Design review of the part built by this model. Coordinates are the model's own, in mm. A direction names the side the tool comes from. Round coordinates to 2 decimals unless told otherwise and drop trailing zeros. Order: outer loops, then holes, each group sorted by start corner. A loop starts at its lowest first (then second) coordinate and runs counter-clockwise, first axis right, second up. Notation, with made-up numbers: (43.25, 85) - (76.25, 85) arc R20 cw to (76.25, 112) - close; hole circle Ø9 at (89, 66). An arc over 180 degrees is marked (long way). Write item = value, one per line.
Autodesk Fusion 360 part; units mm, degrees
sketch "Sketch4" plane through (0, 0, 0) normal (0, 0, 1) x (1, 0, 0)
  line L0 (-17.0224, 4.5069) -> (-7.2135, 4.5755)
  line L1 (-6.882, 4.6055) -> (-0.9889, 5.6389)
  line L2 (-18, 0) -> (-17.9997, 1.25) construction
  line L3 (-17.9997, 1.25) -> (-18.0154, 3.5)
  line L4 (-18, 0) -> (-18, -0.25) construction
  line L5 (-18, -0.25) -> (-3.9671, -0.25)
  line L6 (-17.9997, 1.25) -> (-3.7746, 1.2463)
  arc A0 (2.7555, 5.0182) -> (-0.9889, 5.6389) centre (0, 0) ccw
  arc A1 (-3.9671, -0.25) -> (-3.7746, 1.2463) centre (0, 0) ccw
  line L7 (-18, -0.25) -> (-18, -10)
  line L8 (-15, -13) -> (9, -13)
  line L9 (12, -10) -> (12, -1.8332)
  line L10 (10.444, 0.7965) -> (2.7555, 5.0182)
  arc A2 (-7.2135, 4.5755) -> (-6.882, 4.6055) centre (-7.2274, 6.5754) ccw
  arc A3 (-7.2135, 4.5755) -> (-6.882, 4.6055) centre (-7.2274, 6.5754) ccw
  arc A4 (12, -1.8332) -> (10.444, 0.7965) centre (9, -1.8332) ccw
  arc A5 (9, -13) -> (12, -10) centre (9, -10) ccw
  arc A6 (-18, -10) -> (-15, -13) centre (-15, -10) ccw
  arc A7 (-17.0224, 4.5069) -> (-18.0154, 3.5) centre (-17.0154, 3.507) ccw
  point P0 (-18.0224, 4.4999)
  dimension "d18" = 7.95
  dimension "d22" = 18
  dimension "d24" = 4.5
  dimension "d26" = 1.25
  dimension "d27" = 0.25
  dimension "d28" = 2
  dimension "d29" = 3
  dimension "d30" = 3
  dimension "d31" = 1
  dimension "d56" = 1.75
extrude "Extrude2" add sketch "Sketch4" along normal blind 10 makes body 1
sketch "Sketch5" plane through (-0.0323, 4.6256, 0) normal (-0.007, 1, 0) x (-1, -0.007, 0)
  line L0 (7.1813, 0) -> (16.9905, 0)
  line L1 (16.9905, 0) -> (16.9905, 10)
  line L2 (16.9905, 10) -> (7.1813, 10)
  line L3 (7.1813, 10) -> (7.1813, 0)
  line L4 (12.0859, 10) -> (12.0859, 0) construction
  line L5 (16.9905, 5) -> (7.1813, 5) construction
hole "Hole2" at (-12.1179, 4.5412, 5) direction (0.007, -1, 0) diameter 3 end through all counterbore diameter 6 counterbore depth 2 bodies 1 1
sketch "Sketch6" plane through (0, 0, 10) normal (0, 0, 1) x (-1, 0, 0)
  line L0 (7.2135, -4.5755) -> (17.0224, -4.5069)
  arc A0 (17.0224, -4.5069) -> (18.0154, -3.5) centre (17.0154, -3.507) ccw
  line L1 (18.0154, -3.5) -> (17.9997, -1.25)
  line L2 (17.9997, -1.25) -> (3.7746, -1.2463)
  arc A1 (3.9671, 0.25) -> (3.7746, -1.2463) centre (0, 0) ccw
  line L3 (3.9671, 0.25) -> (18, 0.25)
  line L4 (18, 0.25) -> (18, 10)
  arc A2 (18, 10) -> (15, 13) centre (15, 10) ccw
  line L5 (15, 13) -> (-9, 13)
  arc A3 (-9, 13) -> (-12, 10) centre (-9, 10) ccw
  line L6 (-12, 10) -> (-12, 1.8332)
  arc A4 (-12, 1.8332) -> (-10.444, -0.7965) centre (-9, 1.8332) ccw
  line L7 (-10.444, -0.7965) -> (-2.7555, -5.0182)
  arc A5 (-2.7555, -5.0182) -> (0.9889, -5.6389) centre (0, 0) ccw
  line L8 (0.9889, -5.6389) -> (6.882, -4.6055)
  arc A6 (7.2135, -4.5755) -> (6.882, -4.6055) centre (7.2274, -6.5754) ccw
  line L9 (0, 0) -> (0, 3.975) construction
  line L10 (0, 3.975) -> (-12, 3.975) construction
  line L11 (-12, 3.975) -> (-12, 12.975) construction
  line L12 (-12, 8.475) -> (18, 8.475) construction
  line L13 (0, 3.975) -> (0, 13) construction
  line L14 (7, 8.475) -> (7, 6.4233) construction
  point P0 (-7, 8.475)
  point P1 (7, 8.475)
  dimension "d39" = 9
  dimension "d54" = 14
  dimension "d55" = 7
hole "Hole3" at (7, -8.475, 10) direction (0, 0, -1) diameter 3 end through all counterbore diameter 6 counterbore depth 3 bodies 1 1
hole "Hole4" at (-7, -8.475, 10) direction (0, 0, -1) diameter 3 end through all counterbore diameter 6 counterbore depth 3 bodies 1 1
sketch "Sketch7" plane through (-18, 0, 0) normal (-1, 0, 0) x (0, -1, 0)
  line L0 (0.25, 0) -> (10, 0)
  line L1 (10, 0) -> (10, 10)
  line L2 (10, 10) -> (0.25, 10)
  line L3 (0.25, 10) -> (0.25, 0)
  line L4 (5.125, 10) -> (5.125, 0) construction
  line L5 (10, 5) -> (0.25, 5) construction
  line L6 (6, 7.875) -> (4.25, 7.875)
  line L7 (4.25, 7.875) -> (4.25, 2.125)
  line L8 (4.25, 2.125) -> (6, 2.125)
  line L9 (6, 2.125) -> (6, 7.875)
  line L10 (6, 7.875) -> (4.25, 2.125) construction
  line L11 (4.25, 7.875) -> (6, 2.125) construction
  point P0 (5.125, 5)
  dimension "d50" = 1.75
  dimension "d51" = 5.75
extrude "Extrude3" cut sketch "Sketch7" against normal blind 8.81 contours L6 L7 L8 L9 bodies 1
copy_body "Body->Comp1" bodies 1 removing the originals makes body 2 in component "Guide Rail Clamp 1st Direction"
component "Guide Rail Clamp 1st Direction" placed x (1, 0, 0) y (0, 1, 0) z (0, 0, 1) at (0, 0, 0)
Item 1: The part is to be moulded in two halves that separate along Y. For faces 1 (the face through (8.33, -9.17, 3.45)), 2 (the face through (12, -6, 5)), 3 (the face through (11.14, -12.1, 4.93)), say which applies: +Y half, -Y half, draft (parallel to the pull), parting line (faces both ways), or undercut.
Data:
face_1 = undercut
face_2 = draft
face_3 = -Y half
Item 2: For faces 4 (the face through (-11.445, -9.545, 6.386)), 5 (the face through (-10, -0.25, 5)), 6 (the face through (-7.132, -5.478, 8.479)), list the 3-axis set-ups (+Z, -Z, +X, -X, +Y, -Y) from which the entire face can be reached by the end or side of a thin tool; tool diameter is ignored.
Data:
face_4 = none
face_5 = +Z, -Z, -X
face_6 = +Z
Item 3: Take a section at A-A, the plane x = 7. State the section outline as (y, z) points (3 decimals).
Data:
outline = (-13, 0) - (-9.975, 0) - (-9.975, 7) - (-11.475, 7) - (-11.475, 10) - (-13, 10) - close; (-6.975, 0) - (2.688, 0) - (2.688, 10) - (-5.475, 10) - (-5.475, 7) - (-6.975, 7) - close
Item 4: Take a section at D-D, the plane x = 2. State the section outline as (y, z) points.
Data:
outline = (-13, 0) - (-3.44, 0) - (-3.44, 10) - (-13, 10) - close; (3.44, 0) - (5.36, 0) - (5.36, 10) - (3.44, 10) - close
Item 5: Insertion check: P1, Ø0.5, axis at x = -12, y = -5.5, coming from the -Z side; P2, Ø1.4, axis at y = -5.5, z = 6, coming from the -X side; P3, Ø3.5, axis at x = 7, y = -8.475, coming from the +Z side; P4, Ø3, axis at x = -14.5, z = 3.5, coming from the +Y side. Each pin has a flat end and moves straight along its axis. Give the tip position at first contact, or say it passes through.
Data:
P1 = 0
P2 = -18
P3 = 7
P4 = 4.53
Item 6: For line 1 along Y through (x, z) = (-14.5, 6); line 2 along Y through (x, z) = (-4.5, 1.5); line 3 along X through (y, z) = (-3.5, 4), list the stretches that pass through material, from the lowest coordinate up. Write a range as [from, to].
Data:
line_1 = [-13, -6], [-4.25, -0.25], [1.25, 2.52]
line_2 = [-13, -0.25], [1.25, 5.02]
line_3 = [-18, -13.18], [-10.94, -1.88], [1.88, 12]
Item 7: Take a section at B-B, the plane z = 9. Count the separate pieces of the cut face and the enclosed holes in it, and give its area (3 significant figures).
Data:
separate_pieces = 1
enclosed_holes = 2
area = 383 mm2
